```python
from build123d import *

# Parameters (mm, degrees)
SKETCH1_W           = 40
SKETCH1_H           = 40
BOSS_EXTRUDE1_DEPTH = 40
SKETCH2_W           = 25
SKETCH2_H           = 33
CUT_EXTRUDE1_DEPTH  = 62.5
SKETCH3_R           = 8.5
CUT_EXTRUDE2_DEPTH  = 62.5


with BuildPart() as part:
    # Sketch1 → Boss-Extrude1 (new body)
    with BuildSketch(Plane.XY):
        Rectangle(SKETCH1_W, SKETCH1_H)
    extrude(amount=-BOSS_EXTRUDE1_DEPTH)

    # Sketch2 → Cut-Extrude1 (cut)
    with BuildSketch(Plane(origin=(20, 0, 0), x_dir=(0, 0, -1), z_dir=(1, 0, 0))):
        with Locations((17.5, 3.5)):
            Rectangle(SKETCH2_W, SKETCH2_H)
    extrude(amount=-CUT_EXTRUDE1_DEPTH, mode=Mode.SUBTRACT)

    # Sketch3 → Cut-Extrude2 (cut)
    with BuildSketch(Plane.XY):
        with Locations((0, 2.994290039)):
            Circle(SKETCH3_R)
    extrude(amount=-CUT_EXTRUDE2_DEPTH, mode=Mode.SUBTRACT)


solid = part.part
```
CAD build for the part. Positions are in the model's coordinates, mm. A direction names the side the tool comes from. Round coordinates to 2 decimals unless told otherwise and drop trailing zeros. Order: outer loops, then holes, each group sorted by start corner. A loop starts at its lowest first (then second) coordinate and runs counter-clockwise, first axis right, second up. Notation, with made-up numbers: (43.5, 47.5) -> (66.5, 47.5) arc R35 ccw to (66.5, 80.5) -> close; hole circle Ø3 at (79, 27). An arc over 180 degrees is marked (long way). Write item = value, one per line.
(1) Cut at A-A (y = -7.5). Write the cut outline in (x, z), plus the area to 3 significant figures.
Answers follow:
outline = (-20, -40) -> (20, -40) -> (20, -30) -> (-20, -30) -> close; (-20, -5) -> (20, -5) -> (20, 0) -> (-20, 0) -> close
area = 600 mm²
(2) Drill centre lines: L1, parallel to Y at x = 0, z = -32; L2, parallel to Z at x = 10.5, y = 4; L3, parallel to Y at x = 16, z = -20.5. Where is each one in solid material? Low to high.
Answers follow:
L1 = -20 to -5.51, 11.49 to 20
L2 = -40 to -30, -5 to 0
L3 = -20 to -13
(3) Flat gauge pins, fed straight in: P1, Ø12.5, axis at x = 6.5, z = -14.5, coming from the +Y side; P2, Ø8, axis at y = -0.5, z = -25, coming from the +X side; P3, Ø12, axis at y = -12.5, z = -8, coming from the -X side. Where does each tip first touch, or does it go through?
Answers follow:
P1 = -13
P2 = through
P3 = -20
(4) Pull direction Y, two halves, no side cores. Call faces 3 (the flat face through (0, -13, -17)), 4 (the cylindrical face through (-6.3, 8.7, -2.5)), 5 (the cylindrical face through (-6.3, 8.7, -34.9)), 6 (the flat face through (20, -14, -24)): +Y half, -Y half, draft (parallel to the pull), parting line (faces both ways), or undercut.
Answers follow:
face_3 = +Y half
face_4 = undercut
face_5 = undercut
face_6 = draft
(5) Cut at C-C (x = -13.5). Write the cut outline in (y, z).
Answers follow:
outline = (-20, -40) -> (20, -40) -> (20, -30) -> (-13, -30) -> (-13, -5) -> (20, -5) -> (20, 0) -> (-20, 0) -> close
(6) Cut at D-D (z = -32.5). Write the cut outline in (x, y), plus the area to 3 significant figures.
Answers follow:
outline = (-20, -20) -> (20, -20) -> (20, 20) -> (-20, 20) -> close; hole circle Ø17 at (0, 2.99)
area = 1,370 mm²
(7) Cut at B-B (x = 0). Write the cut outline in (y, z), plus the area to 3 significant figures.
Answers follow:
outline = (-20, -40) -> (-5.51, -40) -> (-5.51, -30) -> (-13, -30) -> (-13, -5) -> (-5.51, -5) -> (-5.51, 0) -> (-20, 0) -> close; (11.49, -40) -> (20, -40) -> (20, -30) -> (11.49, -30) -> close; (11.49, -5) -> (20, -5) -> (20, 0) -> (11.49, 0) -> close
area = 520 mm²
(8) 3-axis set-ups, long thin cutter, end or side, ignore diameter. For faces 1 (the flat face through (5, 11, -30)), 2 (the flat face through (0, 20, -2)): which of +Z, -Z, +X, -X, +Y, -Y reach the whole face in a straight line?
Answers follow:
face_1 = +X, -X, +Y
face_2 = +Z, -Z, +X, -X, +Y
